```python
from build123d import *

# Parameters (mm, degrees)
BOSS_EXTRUDE1_DEPTH                 = 4
BOSS_EXTRUDE2_DEPTH                 = 7.5
CUT_EXTRUDE1_DEPTH                  = 3.5
F_8_0_199_DIAMETER_HOLE1_AT_2_COUNT = 2
F_8_0_199_DIAMETER_HOLE1_AT_2_PITCH = 15
BOSS_EXTRUDE3_REACH                 = 9.5
BOSS_EXTRUDE3_DIRECTION_2_REACH     = 9.5
CUT_EXTRUDE2_DEPTH                  = 3.5
CUT_EXTRUDE2_DEPTH_BACK             = 8
F_8_0_199_DIAMETER_HOLE2_D          = 5.0546
F_8_0_199_DIAMETER_HOLE2_DEPTH      = 11.481444958
F_8_0_199_DIAMETER_HOLE2_TIP        = 1.518555042


with BuildPart() as part:
    # Sketch1 → Boss-Extrude1 (new body, symmetric)
    with BuildSketch(Plane.XY):
        with BuildLine():
            Line((-76, 17.5), (-76, 0))
            Line((-76, 0), (-76, -17.5))
            Line((-76, -17.5), (-72.163391169, -17.5))
            Line((-72.163391169, -17.5), (-68.04053957, -17.5))
            ThreePointArc((-68.04053957, -17.5), (-69.699186267, -8.81977657), (-70.255, 0))
            ThreePointArc((-70.255, 0), (-69.699186267, 8.81977657), (-68.04053957, 17.5))
            Line((-68.04053957, 17.5), (-70.255, 17.5))
            Line((-70.255, 17.5), (-76, 17.5))
        make_face()
        with BuildLine():
            Line((-68.04053957, -17.5), (-72.163391169, -17.5))
            ThreePointArc((-72.163391169, -17.5), (0, -74.255), (72.163391169, -17.5))
            Line((72.163391169, -17.5), (68.04053957, -17.5))
            ThreePointArc((68.04053957, -17.5), (0, -70.255), (-68.04053957, -17.5))
        make_face()
        with BuildLine():
            Line((68.04053957, -17.5), (72.163391169, -17.5))
            Line((72.163391169, -17.5), (76, -17.5))
            Line((76, -17.5), (76, 0))
            Line((76, 0), (76, 17.5))
            Line((76, 17.5), (70.255, 17.5))
            Line((70.255, 17.5), (68.04053957, 17.5))
            ThreePointArc((68.04053957, 17.5), (69.699186267, 8.81977657), (70.255, 0))
            ThreePointArc((70.255, 0), (69.699186267, -8.81977657), (68.04053957, -17.5))
        make_face()
    extrude(amount=BOSS_EXTRUDE1_DEPTH, both=True)

    # Sketch1_5 → Boss-Extrude2 (add, symmetric)
    with BuildSketch(Plane.XY):
        with BuildLine():
            Line((-76, 17.5), (-76, 0))
            Line((-76, 0), (-76, -17.5))
            Line((-76, -17.5), (-72.163391169, -17.5))
            Line((-72.163391169, -17.5), (-68.04053957, -17.5))
            ThreePointArc((-68.04053957, -17.5), (-69.699186267, -8.81977657), (-70.255, 0))
            ThreePointArc((-70.255, 0), (-69.699186267, 8.81977657), (-68.04053957, 17.5))
            Line((-68.04053957, 17.5), (-70.255, 17.5))
            Line((-70.255, 17.5), (-76, 17.5))
        make_face()
        with BuildLine():
            Line((68.04053957, -17.5), (72.163391169, -17.5))
            Line((72.163391169, -17.5), (76, -17.5))
            Line((76, -17.5), (76, 0))
            Line((76, 0), (76, 17.5))
            Line((76, 17.5), (70.255, 17.5))
            Line((70.255, 17.5), (68.04053957, 17.5))
            ThreePointArc((68.04053957, 17.5), (69.699186267, 8.81977657), (70.255, 0))
            ThreePointArc((70.255, 0), (69.699186267, -8.81977657), (68.04053957, -17.5))
        make_face()
    extrude(amount=BOSS_EXTRUDE2_DEPTH, both=True)

    # Sketch2 → Cut-Extrude1 (cut, symmetric)
    with BuildSketch(Plane.ZY.offset(-70.255)):
        Polygon((0, 2.332715091), (4.475, 4.916357545), (4.475, 10.083642455), (0, 12.667284909), (-4.475, 10.083642455), (-4.475, 4.916357545), align=None)
        Polygon((0, -12.667284909), (4.475, -10.083642455), (4.475, -4.916357545), (0, -2.332715091), (-4.475, -4.916357545), (-4.475, -10.083642455), align=None)
    cut_extrude1 = extrude(amount=CUT_EXTRUDE1_DEPTH, both=True, mode=Mode.SUBTRACT)

    # Sketch4 → 8 _0.199_ Diameter Hole1 (revolve, cut)
    with BuildSketch(Plane(origin=(76, 7.5, 0), x_dir=(0, 0, -1), z_dir=(0, 1, 0))):
        Polygon((0, 0), (0, 10.71), (2.5273, 9.191444958), (2.5273, 0), align=None)
    f_8_0_199_diameter_hole1 = revolve(axis=Axis((82.35, 7.5, 0), (-1, 0, 0)), mode=Mode.SUBTRACT)

    # 8 _0.199_ Diameter Hole1 at 2: 8 _0.199_ Diameter Hole1 ×2
    with Locations(*[(0, -i * F_8_0_199_DIAMETER_HOLE1_AT_2_PITCH, 0) for i in range(1, F_8_0_199_DIAMETER_HOLE1_AT_2_COUNT)]):
        add(f_8_0_199_diameter_hole1, mode=Mode.SUBTRACT)

    # Mirror1: 8 _0.199_ Diameter Hole1, Cut-Extrude1 across plane
    add(f_8_0_199_diameter_hole1.mirror(Plane(origin=(0, 0, 0), x_dir=(0, 0, 1), z_dir=(1, 0, 0))), mode=Mode.SUBTRACT)
    add(cut_extrude1.mirror(Plane(origin=(0, 0, 0), x_dir=(0, 0, 1), z_dir=(1, 0, 0))), mode=Mode.SUBTRACT)

    # Mirror1 copy 1 sketch → Mirror1 copy 1 (revolve, cut)
    with BuildSketch(Plane(origin=(-76, -7.5, 0), x_dir=(0, 0, -1), z_dir=(0, 1, 0))):
        Polygon((0, 0), (0, -10.71), (2.5273, -9.191444958), (2.5273, 0), align=None)
    revolve(axis=Axis((-82.35, -7.5, 0), (-1, 0, 0)), mode=Mode.SUBTRACT)

    # Boss-Extrude3: up to this face of the body (flat: up to its plane)
    boss_extrude3_end = Plane(part.part.faces().sort_by_distance((-72.727295349, 0, 7.5))[0])
    # Sketch5 → Boss-Extrude3 (add, up to the picked face)
    with BuildSketch(Plane.XY, mode=Mode.PRIVATE) as boss_extrude3_sk1:
        with BuildLine():
            Line((47.5, -57.074994744), (47.5, -74.255))
            Line((47.5, -74.255), (32.5, -74.255))
            Line((32.5, -74.255), (32.5, -62.285752986))
            ThreePointArc((32.5, -62.285752986), (36.825261363, -59.830302946), (40.96596148, -57.074994744))
            Line((40.96596148, -57.074994744), (47.5, -57.074994744))
        make_face()
    boss_extrude3_tool1 = split(extrude(boss_extrude3_sk1.sketch, amount=BOSS_EXTRUDE3_REACH, mode=Mode.PRIVATE), bisect_by=boss_extrude3_end, keep=Keep.BOTH, mode=Mode.PRIVATE)
    add(boss_extrude3_tool1.solids().sort_by_distance((40.456136, -66.339152, 0))[0])
    # Sketch5 → Boss-Extrude3 (add, up to the picked face)
    with BuildSketch(Plane.XY, mode=Mode.PRIVATE) as boss_extrude3_sk2:
        with BuildLine():
            Line((-32.5, -74.255), (-47.5, -74.255))
            Line((-47.5, -74.255), (-47.5, -57.074994744))
            Line((-47.5, -57.074994744), (-40.96596148, -57.074994744))
            ThreePointArc((-40.96596148, -57.074994744), (-36.825261363, -59.830302946), (-32.5, -62.285752986))
            Line((-32.5, -62.285752986), (-32.5, -74.255))
        make_face()
    boss_extrude3_tool2 = split(extrude(boss_extrude3_sk2.sketch, amount=BOSS_EXTRUDE3_REACH, mode=Mode.PRIVATE), bisect_by=boss_extrude3_end, keep=Keep.BOTH, mode=Mode.PRIVATE)
    add(boss_extrude3_tool2.solids().sort_by_distance((-40.456136, -66.339152, 0))[0])

    # Boss-Extrude3 direction 2: up to this face of the body (flat: up to its plane)
    boss_extrude3_direction_2_end = Plane(part.part.faces().sort_by_distance((-72.727295349, 0, -7.5))[0])
    # Sketch5 → Boss-Extrude3 direction 2 (add, up to the picked face)
    with BuildSketch(Plane.XY, mode=Mode.PRIVATE) as boss_extrude3_direction_2_sk1:
        with BuildLine():
            Line((47.5, -57.074994744), (47.5, -74.255))
            Line((47.5, -74.255), (32.5, -74.255))
            Line((32.5, -74.255), (32.5, -62.285752986))
            ThreePointArc((32.5, -62.285752986), (36.825261363, -59.830302946), (40.96596148, -57.074994744))
            Line((40.96596148, -57.074994744), (47.5, -57.074994744))
        make_face()
    boss_extrude3_direction_2_tool1 = split(extrude(boss_extrude3_direction_2_sk1.sketch, amount=-BOSS_EXTRUDE3_DIRECTION_2_REACH, mode=Mode.PRIVATE), bisect_by=boss_extrude3_direction_2_end, keep=Keep.BOTH, mode=Mode.PRIVATE)
    add(boss_extrude3_direction_2_tool1.solids().sort_by_distance((40.456136, -66.339152, 0))[0])
    # Sketch5 → Boss-Extrude3 direction 2 (add, up to the picked face)
    with BuildSketch(Plane.XY, mode=Mode.PRIVATE) as boss_extrude3_direction_2_sk2:
        with BuildLine():
            Line((-32.5, -74.255), (-47.5, -74.255))
            Line((-47.5, -74.255), (-47.5, -57.074994744))
            Line((-47.5, -57.074994744), (-40.96596148, -57.074994744))
            ThreePointArc((-40.96596148, -57.074994744), (-36.825261363, -59.830302946), (-32.5, -62.285752986))
            Line((-32.5, -62.285752986), (-32.5, -74.255))
        make_face()
    boss_extrude3_direction_2_tool2 = split(extrude(boss_extrude3_direction_2_sk2.sketch, amount=-BOSS_EXTRUDE3_DIRECTION_2_REACH, mode=Mode.PRIVATE), bisect_by=boss_extrude3_direction_2_end, keep=Keep.BOTH, mode=Mode.PRIVATE)
    add(boss_extrude3_direction_2_tool2.solids().sort_by_distance((-40.456136, -66.339152, 0))[0])

    # Sketch6 → Cut-Extrude2 (cut, two sides)
    with BuildSketch(Plane(origin=(0, -57.074994744, 0), x_dir=(1, 0, 0), z_dir=(0, 1, 0))) as cut_extrude2_sk:
        Polygon((-37.416357545, -4.475), (-34.832715091, 0), (-37.416357545, 4.475), (-42.583642455, 4.475), (-45.167284909, 0), (-42.583642455, -4.475), align=None)
        Polygon((42.583642455, -4.475), (45.167284909, 0), (42.583642455, 4.475), (37.416357545, 4.475), (34.832715091, 0), (37.416357545, -4.475), align=None)
    extrude(amount=CUT_EXTRUDE2_DEPTH, mode=Mode.SUBTRACT)
    extrude(cut_extrude2_sk.sketch, amount=-CUT_EXTRUDE2_DEPTH_BACK, mode=Mode.SUBTRACT)

    # 8 _0.199_ Diameter Hole2
    with Locations(Plane(origin=(-40, -74.255, 0), x_dir=(0, 0, -1), z_dir=(0, -1, 0))):
        with Locations((0, 0), (0, 80)):
            Hole(F_8_0_199_DIAMETER_HOLE2_D / 2, depth=F_8_0_199_DIAMETER_HOLE2_DEPTH)
            with Locations((0, 0, -(F_8_0_199_DIAMETER_HOLE2_DEPTH + F_8_0_199_DIAMETER_HOLE2_TIP / 2))):  # 118° drill point
                Cone(0, F_8_0_199_DIAMETER_HOLE2_D / 2, F_8_0_199_DIAMETER_HOLE2_TIP, mode=Mode.SUBTRACT)


solid = part.part
```
Build history of the part. All positions in model axes, mm. A direction names the side the tool comes from. Give positions to 0.01 mm unless a question says otherwise; leave off trailing zeros. Loops run counter-clockwise (first coordinate to the right, second up) from the corner with the lowest first, then second, coordinate; pieces in that order, holes last. Notation, with made-up numbers: (62, -7.5) -> (115, -7.5) arc R12 cw to (115, 1.5) -> close; hole circle Ø1 at (-19.5, -13). An arc over 180 degrees is marked (long way). One line per question, with ' | ' between items.
Q1. Drill centre lines: line 1 along Y through (x, z) = (-75.4, 0); line 2 along X through (y, z) = (-0.5, -4); line 3 along X through (y, z) = (12.5, -4.5). Where is each one in solid material? Low to high. Write a range as [from, to].
Filled sheet:
line 1: y = [-17.5, -10.03], [-4.97, 4.97], [10.03, 17.5] | line 2: x = [-76, -70.25], [70.25, 76] | line 3: x = [-76, -69.13], [69.13, 76]
Q2. Pull direction Y, two halves, no side cores. Call faces 4 (the flat face through (-37, -74.255, 0)), 5 (the flat face through (60, -39, -4)), 6 (the flat face through (72, 8, -4.475)): pulls with the +Y half, pulls with the -Y half, needs draft (parallel to the pull), parting line crosses it, or undercut.
Filled sheet:
face 4: pulls with the -Y half | face 5: needs draft | face 6: undercut
Q3. Cut at C-C, the plane x = 64. Write the cut outline in (y, z), plus the area to 3 significant figures.
Filled sheet:
outline: (-37.65, -4) -> (-28.98, -4) -> (-28.98, 4) -> (-37.65, 4) -> close | area: 69.4 mm²
Q4. Cut at B-B, the plane y = -52. Write the cut outline in (x, z).
Filled sheet:
outline: (-53.01, -4) -> (-47.24, -4) -> (-47.24, 4) -> (-53.01, 4) -> close; (47.24, -4) -> (53.01, -4) -> (53.01, 4) -> (47.24, 4) -> close
Q5. Drop flat-ended pins along their axis: pin 1 (2.5 mm diameter, centred on x = -73.5, z = 0.5, fed in from -Y); pin 2 (1.5 mm diameter, centred on x = 6, z = -2, fed in from -Y); pin 3 (6 mm diameter, centred on y = -70, z = 0.5, fed in from +X); pin 4 (1.5 mm diameter, centred on x = -49, z = 5, fed in from -Y). Give the stop position or say it passes through.
Filled sheet:
pin 1: stops at y = -17.5 | pin 2: stops at y = -74.07 | pin 3: stops at x = 47.5 | pin 4: passes through
Q6. Tool access for faces 1 (the cylindrical face through (-63.194, -38.992, 0.056)), 2 (the flat face through (-73.755, -5, 1)), 3 (the flat face through (-40, -61, 4.475)): list every direction of +Z, -Z, +X, -X, +Y, -Y with a clear straight run to the whole face (end or side of a thin tool).
Filled sheet:
face 1: +Z, -Z, -X, -Y | face 2: none | face 3: +Y
Q7. Cut at D-D, the plane y = -19. Write the cut outline in (x, z), plus the area to 3 significant figures.
Filled sheet:
outline: (-71.78, -4) -> (-67.64, -4) -> (-67.64, 4) -> (-71.78, 4) -> close; (67.64, -4) -> (71.78, -4) -> (71.78, 4) -> (67.64, 4) -> close | area: 66.3 mm²
Q8. Cut at A-A, the plane y = -7.5. Write the cut outline in (x, z) (3 decimals).
Filled sheet:
outline: (-76, -7.5) -> (-69.854, -7.5) -> (-69.854, -4.475) -> (-73.755, -4.475) -> (-73.755, -2.527) -> (-76, -2.527) -> close; (-76, 2.527) -> (-73.755, 2.527) -> (-73.755, 4.475) -> (-69.854, 4.475) -> (-69.854, 7.5) -> (-76, 7.5) -> close; (69.854, -7.5) -> (76, -7.5) -> (76, -2.527) -> (73.755, -2.527) -> (73.755, -4.475) -> (69.854, -4.475) -> close; (69.854, 4.475) -> (73.755, 4.475) -> (73.755, 2.527) -> (76, 2.527) -> (76, 7.5) -> (69.854, 7.5) -> close
